Autodesk Inventor part; units mm, degrees
ref_plane "YZ Plane" through (0, 0, 0) normal (1, 0, 0) x (0, 1, 0)
ref_plane "XZ Plane" through (0, 0, 0) normal (0, 1, 0) x (-1, 0, 0)
ref_plane "XY Plane" through (0, 0, 0) normal (0, 0, 1) x (1, 0, 0)
sketch "Skizze1" plane through (0, 0, 0) normal (0, 0, 1) x (1, 0, 0)
  line L0 (-17.5, 0) -> (17.5, 0)
  line L1 (0, -17.5) -> (0, 17.5)
  circle A0 centre (0, 0) radius 12.5
  dimension "d0" = 25
extrude "Extrusion1" add sketch "Skizze1" along normal blind 60
sketch "Skizze2" plane through (0, 0, 60) normal (0, 0, 1) x (1, 0, 0)
  circle A0 centre (0, 0) radius 10.8915
sketch "Skizze3" plane through (0, 0, 0) normal (1, 0, 0) x (0, 1, 0)
  line L0 (12.5, 0) -> (-12.5, 0)
  circle A0 centre (0, 30) radius 12.5
  point P0 (0, 0)
  dimension "d3" = 30
  dimension "d4" = 25
extrude "Extrusion2" add sketch "Skizze3" against normal blind 30
sketch "Skizze4" plane through (0, 0, 0) normal (0, 0, -1) x (-1, 0, 0)
  point P0 (0, 0)
hole "Bohrung1" at (0, 0, 0) direction (0, 0, 1) diameter 17.294 depth 30
hole "Bohrung2" at (0, 0, 60) direction (0, 0, -1) diameter 17.294 depth 30
sketch "Skizze5" plane through (-30, 0, 30) normal (-1, 0, 0) x (0, 0, 1)
  point P0 (-30, 0)
  point P1 (0.0118, -0.0059)
hole "Bohrung3" at (-30, -0.0059, 30.0118) direction (1, 0, 0) diameter 17.294 depth 30
chamfer "Fase1" distance 0.5 angle 45 6 edges at (-12.5, 0, 60) (0, 8.647, 60) (-30, -12.5, 30) (-30, -0.0059, 21.3648) (-12.5, 0, 0) (0, -8.647, 0)
properties part number "Verbindungsstück"
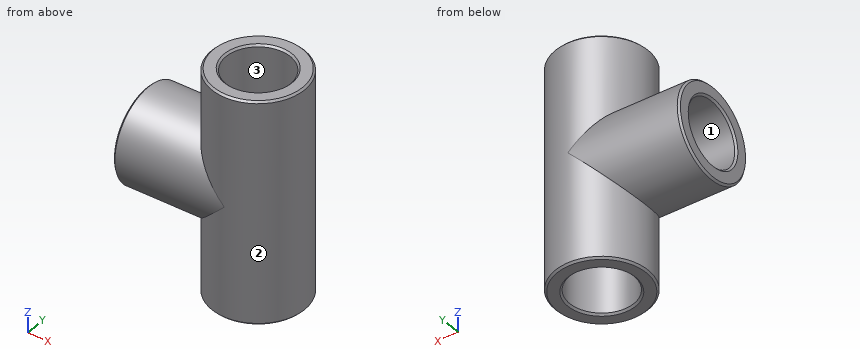
Geometry: final body of the model. Coordinates: model frame, mm. Face numbers are marked on the shaded views. Round coordinates to 2 decimals unless told otherwise and drop trailing zeros. Order: outer loops, then holes, each group sorted by start corner. A loop starts at its lowest first (then second) coordinate and runs counter-clockwise, first axis right, second up. Notation, with made-up numbers: (-24, 35) -> (26, 35) arc R38 ccw to (26, 73) -> close; hole circle Ø5 at (24, 74.25). An arc over 180 degrees is marked (long way). Use CSV: the item, a comma, the result in double quotes. Start each with the question number.
1) First-contact query: pin 1 Ø5 at (y, z) = (-8.5, 26.5) entering from +X; pin 2 Ø6 at (x, z) = (7, 37.5) entering from +Y; pin 3 Ø6 at (x, y) = (-23, -0.5) entering from -Z. Flat tips, straight axial feed; report the tip coordinate or a pass-through.
2) Draft query along X for the marked faces 1, 2 and 3. Return one class per face: +X half, -X half, draft (parallel to the pull), parting line (faces both ways), or undercut.
3) Section B-B (y = 6.25). State how many separate pieces and enclosed holes the cut face has, and give its area (3 significant figures).
4) Section A-A (z = 12). Return the cut outline in (x, y), and give its area (3 significant figures).
5) Material intervals for line 1 along Y through (x, z) = (0, 16); line 2 along X through (y, z) = (0, 18); line 3 along X through (y, z) = (0, 30), sorted ascending. Write a range as from..to.
Returned:
1,pin 1,"stops at x = 10.97"
1,pin 2,"stops at y = 11.84"
1,pin 3,"stops at z = 17.5"
2,face 1,"draft"
2,face 2,"parting line"
2,face 3,"undercut"
3,separate pieces,"3"
3,enclosed holes,"0"
3,area,"708 mm²"
4,outline,"circle Ø25 at (0, 0); hole circle Ø17.29 at (0, 0)"
4,area,"256 mm²"
5,line 1,"y = -12.5..-8.65, 8.65..12.5"
5,line 2,"x = -30..-8.65, 8.65..12.5"
5,line 3,"x = 8.65..12.5"
